Autodesk Inventor part; units mm, degrees
ref_plane "YZ Plane" through (0, 0, 0) normal (1, 0, 0) x (0, 1, 0)
ref_plane "XZ Plane" through (0, 0, 0) normal (0, 1, 0) x (-1, 0, 0)
ref_plane "XY Plane" through (0, 0, 0) normal (0, 0, 1) x (1, 0, 0)
sketch "Szkic1" plane through (0, 0, 0) normal (0, 0, 1) x (1, 0, 0)
  circle A0 centre (0, 16) radius 3
  circle A1 centre (0, -16) radius 3
  line L0 (0, 0) -> (20, 0)
  line L1 (20, 0) -> (20, -42.5)
  line L2 (20, 0) -> (20, 42.5)
  line L3 (20, 0) -> (62.5, 0) construction
  line L4 (20, 42.5) -> (-78, 42.5)
  line L5 (-78, 42.5) -> (-78, -42.5)
  line L6 (-78, -42.5) -> (20, -42.5)
  dimension "d0" = 6
  dimension "d1" = 6
  dimension "d5" = 20
  dimension "d6" = 42.5
  dimension "d7" = 42.5
  dimension "d8" = 90
  dimension "d9" = 98
  dimension "d10" = 85
  dimension "d11" = 90
extrude "Wyciągnięcie proste1" add sketch "Szkic1" along normal blind 3
sketch "Szkic2" plane through (0, 0, 3) normal (0, 0, 1) x (1, 0, 0)
  line L0 (-78, -42.5) -> (20, -42.5)
  line L1 (-10, 42.5) -> (10, 42.5)
  line L2 (10, 42.5) -> (10, -42.5)
  line L3 (10, -42.5) -> (-10, -42.5)
  line L4 (-10, -42.5) -> (-10, 42.5)
  line L5 (-10, 42.5) -> (10, -42.5) construction
  line L6 (10, 42.5) -> (-10, -42.5) construction
  circle A0 centre (-14, 39) radius 1
  circle A1 centre (-14, 39) radius 2.5
  circle A2 centre (-63, 39) radius 2.5
  circle A3 centre (-63, 39) radius 1
  circle A4 centre (-14, -19) radius 2.5
  circle A5 centre (-14, -19) radius 1
  circle A6 centre (-63, -19) radius 2.5
  circle A7 centre (-63, -19) radius 1
  line L7 (10, 42.5) -> (14, 42.5)
  line L8 (14, 42.5) -> (14, -42.5)
  line L9 (14, -42.5) -> (10, -42.5)
  line L10 (10, -42.5) -> (10, 42.5)
  point P0 (0, 0)
  dimension "d14" = 20
  dimension "d15" = 2
  dimension "d16" = 1.5
  dimension "d19" = 49
  dimension "d22" = 58
  dimension "d25" = 4
extrude "Wyciągnięcie proste2" add sketch "Szkic2" along normal blind 2 contours A1 | A2 | A4 | A6
extrude "Wyciągnięcie proste3" cut sketch "Szkic2" against normal blind 3 contours A0 | A3 | A5 | A7
sketch "Szkic4" plane through (0, 0, 3) normal (0, 0, 1) x (1, 0, 0)
  line L0 (-78, 42.5) -> (-78, -42.5)
  line L1 (-78, -42.5) -> (-68, -42.5)
  line L2 (-68, -42.5) -> (-68, -40.5)
  line L3 (-68, -40.5) -> (-78, -40.5)
  line L4 (-78, -40.5) -> (-78, -42.5)
  line L5 (-78, 42.5) -> (-68, 42.5)
  line L6 (-68, 42.5) -> (-68, 40.5)
  line L7 (-68, 40.5) -> (-78, 40.5)
  line L8 (-78, 40.5) -> (-78, 42.5)
  point P0 (0, 0)
  dimension "d31" = 10
  dimension "d32" = 2
  dimension "d33" = 10
  dimension "d34" = 2
extrude "Wyciągnięcie proste4" add sketch "Szkic4" along normal blind 42.5
sketch "Szkic5" plane through (0, 0, 45.5) normal (0, 0, 1) x (1, 0, 0)
  line L0 (-78, -42.5) -> (20, -42.5)
  line L1 (20, 42.5) -> (-78, 42.5)
  line L2 (-78, -42.5) -> (-33, -42.5)
  line L3 (-33, -42.5) -> (-33, 42.5)
  line L4 (-33, 42.5) -> (-78, 42.5)
  line L5 (-78, 42.5) -> (-78, -42.5)
  line L6 (-51.815, 0) -> (-51.815, 29.5)
  line L7 (-51.815, 29.5) -> (-51.815, -29.5)
  line L8 (-41.815, -29.5) -> (-61.815, -29.5) construction
  line L9 (-41.815, -27.5) -> (-61.815, -27.5)
  line L10 (-61.815, -31.5) -> (-41.815, -31.5)
  arc A0 (-41.815, -31.5) -> (-41.815, -27.5) centre (-41.815, -29.5) ccw
  arc A1 (-61.815, -27.5) -> (-61.815, -31.5) centre (-61.815, -29.5) ccw
  line L11 (-41.815, 29.5) -> (-61.815, 29.5) construction
  line L12 (-41.815, 31.5) -> (-61.815, 31.5)
  line L13 (-61.815, 27.5) -> (-41.815, 27.5)
  arc A2 (-41.815, 27.5) -> (-41.815, 31.5) centre (-41.815, 29.5) ccw
  arc A3 (-61.815, 31.5) -> (-61.815, 27.5) centre (-61.815, 29.5) ccw
  point P0 (0, 0)
  dimension "d37" = 45
  dimension "d38" = 29.5
  dimension "d39" = 59
  dimension "d40" = 10
  dimension "d41" = 4
  dimension "d42" = 4
extrude "Wyciągnięcie proste5" add sketch "Szkic5" against normal blind 1.5
sketch "Szkic6" plane through (0, 0, 0) normal (0, 0, -1) x (-1, 0, 0)
  circle A0 centre (-18, 0) radius 2
  circle A1 centre (-18, 0) radius 1
  line L0 (-18, 0) -> (53.3, 0)
  line L1 (53.3, 0) -> (53.3, 18)
  line L2 (53.3, 0) -> (53.3, -18)
  circle A2 centre (53.3, -18) radius 1
  circle A3 centre (53.3, -18) radius 2
  circle A4 centre (53.3, 18) radius 1
  circle A5 centre (53.3, 18) radius 2
  arc A6 (53.3, 14) -> (53.3, -14) centre (53.3, 0) ccw
  line L3 (53.3, -14) -> (78, -18.3553)
  line L4 (78, 40.5) -> (78, -40.5)
  line L5 (53.3, -14) -> (78.381, -14) construction
  line L6 (53.3, 14) -> (78, 18.3553)
  line L7 (53.3, 14) -> (78.381, 14) construction
  line L8 (78, 18.3553) -> (78, -18.3553)
  point P0 (0, 0)
  dimension "d45" = 2
  dimension "d46" = 71.3
  dimension "d47" = 18
  dimension "d48" = 18
  dimension "d49" = 2
  dimension "d50" = 4
  dimension "d51" = 2
  dimension "d52" = 4
  dimension "d53" = 14
  dimension "d54" = 10
  dimension "d55" = 10
extrude "Wyciągnięcie proste6" add sketch "Szkic6" along normal blind 8 contours A0 | A5 | A3
extrude "Wyciągnięcie proste7" cut sketch "Szkic6" against normal blind 3 contours A6 L1 L0 | L0 L2 A6 | L1 L6 L4 L3 L2
properties part number "RP4_LidarHolderv3"
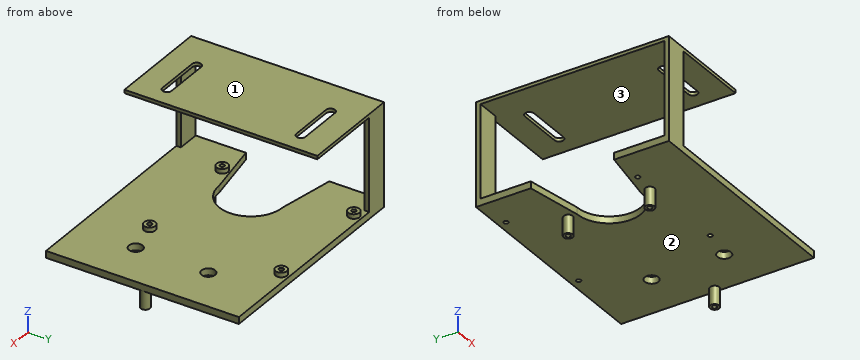
Here's how the part is built. I have some questions about the finished solid (model axes, mm). Face numbers are marked on the shaded views. Give positions to 0.01 mm unless a question says otherwise; leave off trailing zeros. Loops run counter-clockwise (first coordinate to the right, second up) from the corner with the lowest first, then second, coordinate; pieces in that order, holes last. Notation, with made-up numbers: M 16.25,17 L 25.25,17 A22 ccw 25.25,45 Z; hole C 84,46 d6. An arc over 180 degrees is marked long. Return JSON: item names as keys, results as strings.
Item 1: Thinking about a two-plate mould opening in Z: for the marked faces 1, 2 and 3, which applies, released by +Z, released by -Z, zero draft, split by the parting line, or undercut?
A:
{"face 1": "released by +Z", "face 2": "released by -Z", "face 3": "undercut"}
Item 2: I'm going to push flat-ended pins straight in: pin 1 Ø1.2 at (y, z) = (10.5, 45) entering from +X; pin 2 Ø0.6 at (y, z) = (-42, 18) entering from +X; pin 3 Ø5 at (x, y) = (7.5, -29.5) entering from +Z. Where does each tip first touch, or does it pass through?
A:
{"pin 1": "stops at x = -33", "pin 2": "stops at x = -68", "pin 3": "stops at z = 3"}
Item 3: Please list where these lines run through material, in increasing order: line 1 (Y direction, x = -14, z = 3.5); line 2 (Y direction, x = -53.3, z = -2.5); line 3 (Y direction, x = -71, z = 41).
A:
{"line 1": "y = -21.5 to -20, -18 to -16.5, 36.5 to 38, 40 to 41.5", "line 2": "y = -20 to -19, -17 to -16, 16 to 17, 19 to 20", "line 3": "y = -42.5 to -40.5, 40.5 to 42.5"}
Item 4: Imagine slicing it at B-B on z = 42. List the corners of the cut face in (x, y) for me.
A:
{"outline": "M -78,-42.5 L -68,-42.5 L -68,-40.5 L -78,-40.5 Z; M -78,40.5 L -68,40.5 L -68,42.5 L -78,42.5 Z"}
Item 5: Imagine slicing it at C-C on x = 0. List the corners of the cut face in (y, z) for me.
A:
{"outline": "M -42.5,0 L -19,0 L -19,3 L -42.5,3 Z; M -13,0 L 13,0 L 13,3 L -13,3 Z; M 19,0 L 42.5,0 L 42.5,3 L 19,3 Z"}
Item 6: Imagine slicing it at A-A on y = -35. List the corners of the cut face in (x, z) for me, then the cut area to 4 significant figures.
A:
{"outline": "M -78,0 L 20,0 L 20,3 L -78,3 Z; M -78,44 L -33,44 L -33,45.5 L -78,45.5 Z", "area": "361.5 mm^2"}
Item 7: Imagine slicing it at D-D on x = -59. List the corners of the cut face in (y, z) for me, then the cut area to 3 significant figures.
A:
{"outline": "M -42.5,0 L -15.01,0 L -15.01,3 L -42.5,3 Z; M -42.5,44 L -31.5,44 L -31.5,45.5 L -42.5,45.5 Z; M -27.5,44 L 27.5,44 L 27.5,45.5 L -27.5,45.5 Z; M 15.01,0 L 42.5,0 L 42.5,3 L 15.01,3 Z; M 31.5,44 L 42.5,44 L 42.5,45.5 L 31.5,45.5 Z", "area": "280 mm^2"}
